Can you work these out from the model? Positions are in its coordinate system, mm. Coordinates: 2 decimals unless noted, no trailing zeros. Order: outer loops, then holes, each group sorted by start corner. A loop starts at its lowest first (then second) coordinate and runs counter-clockwise, first axis right, second up. Notation, with made-up numbers: (9.5, 50) -> (38.5, 50) arc R31 cw to (38.5, 75) -> close; hole circle Ø8 at (75, 76). An arc over 180 degrees is marked (long way). Answer in a Markdown table with one row per item.
```python
from build123d import *

# Parameters (mm, degrees)
F1_DEPTH = 50.8
F2_R     = 127
F3_R     = 127
F4_R     = 127
F5_R     = 127


with BuildPart() as f1:
    # F0 (on Front) → F1 (new body)
    with BuildSketch(Plane.XZ):
        with BuildLine():
            Line((101.6, 317.5), (254, 317.5))
            ThreePointArc((254, 317.5), (0, 571.5), (-254, 317.5))
            Line((-254, 317.5), (-101.6, 317.5))
            ThreePointArc((-101.6, 317.5), (0, 419.1), (101.6, 317.5))
        make_face()
        with BuildLine():
            ThreePointArc((254, -317.5), (184.7032192794, 0), (254, 317.5))
            Line((254, 317.5), (101.6, 317.5))
            ThreePointArc((101.6, 317.5), (0, 215.9), (-101.6, 317.5))
            Line((-101.6, 317.5), (-254, 317.5))
            ThreePointArc((-254, 317.5), (-184.7032192794, 0), (-254, -317.5))
            Line((-254, -317.5), (-101.6, -317.5))
            ThreePointArc((-101.6, -317.5), (0, -215.9), (101.6, -317.5))
            Line((101.6, -317.5), (254, -317.5))
        make_face()
        with BuildLine():
            ThreePointArc((-254, -317.5), (0, -571.5), (254, -317.5))
            Line((254, -317.5), (101.6, -317.5))
            ThreePointArc((101.6, -317.5), (0, -419.1), (-101.6, -317.5))
            Line((-101.6, -317.5), (-254, -317.5))
        make_face()
    extrude(amount=F1_DEPTH)

    # F2
    f2_edges = [f1.edges().sort_by_distance(p)[0] for p in [
        (-254, -25.4, -317.5),
    ]]
    fillet(f2_edges, radius=F2_R)

    # F3
    f3_edges = [f1.edges().sort_by_distance(p)[0] for p in [
        (-254, -25.4, 317.5),
    ]]
    fillet(f3_edges, radius=F3_R)

    # F4
    f4_edges = [f1.edges().sort_by_distance(p)[0] for p in [
        (254, -25.4, 317.5),
    ]]
    fillet(f4_edges, radius=F4_R)

    # F5
    f5_edges = [f1.edges().sort_by_distance(p)[0] for p in [
        (254, -25.4, -317.5),
    ]]
    fillet(f5_edges, radius=F5_R)


solid = f1.part
```
(1) We'd pull the mould along Z, two halves only. Please class faces 1 (the cylindrical face through (-22.025, -25.044, 416.684)), 2 (the cylindrical face through (-4.97, -25.04, -571.45)), 3 (the flat face through (-4, 0, 8)): +Z half, -Z half, draft (parallel to the pull), parting line (faces both ways), or undercut.
Response values:
| item | result |
|---|---|
| face 1 | undercut |
| face 2 | -Z half |
| face 3 | draft |
(2) Suppose I cut it at C-C (x = -208.5). Please give me the cut outline in (y, z).
Response values:
| item | result |
|---|---|
| outline | (-50.8, -462.56) -> (0, -462.56) -> (0, -188.94) -> (-50.8, -188.94) -> close; (-50.8, 188.94) -> (0, 188.94) -> (0, 462.56) -> (-50.8, 462.56) -> close |
(3) Suppose I cut it at D-D (y = -42). Count the separate pieces of the cut face and the enclosed holes in it, and give its area (3 significant figures).
Response values:
| item | result |
|---|---|
| separate pieces | 1 |
| enclosed holes | 2 |
| area | 401,000 mm2 |
(4) Suppose I cut it at B-B (z = 227). Please give me the cut outline in (x, y), and give its area (3 significant figures).
Response values:
| item | result |
|---|---|
| outline | (-219.3, -50.8) -> (-46.18, -50.8) -> (-46.18, 0) -> (-219.3, 0) -> close; (46.18, -50.8) -> (219.3, -50.8) -> (219.3, 0) -> (46.18, 0) -> close |
| area | 17,600 mm2 |
(5) Suppose I cut it at A-A (x = 0). Please give me the cut outline in (y, z).
Response values:
| item | result |
|---|---|
| outline | (-50.8, -571.5) -> (0, -571.5) -> (0, -419.1) -> (-50.8, -419.1) -> close; (-50.8, -215.9) -> (0, -215.9) -> (0, 215.9) -> (-50.8, 215.9) -> close; (-50.8, 419.1) -> (0, 419.1) -> (0, 571.5) -> (-50.8, 571.5) -> close |
(6) I need wall thicknesses on line 1 (X direction, y = -14, z = 317); line 2 (X direction, y = -10, z = 317.5); line 3 (Z direction, x = -76, y = -31). Which ranges of each line are inside material? Lowest first, please. Write a range as [from, to].
Response values:
| item | result |
|---|---|
| line 1 | [-250.07, -101.6], [101.6, 250.07] |
| line 2 | [-250.16, -101.6], [101.6, 250.16] |
| line 3 | [-559.86, -384.93], [-250.07, 250.07], [384.93, 559.86] |
(7) Will these pins go through, and if not, where does the flat tip stop? pin 1 Ø1.5 at (x, y) = (86, -15.5) entering from +Z; pin 2 Ø3 at (x, y) = (-124.5, -6) entering from -Z; pin 3 Ø4 at (y, z) = (-21, -263.5) entering from -X.
Response values:
| item | result |
|---|---|
| pin 1 | z = 556.77 |
| pin 2 | z = -539.73 |
| pin 3 | x = -232.45 |
